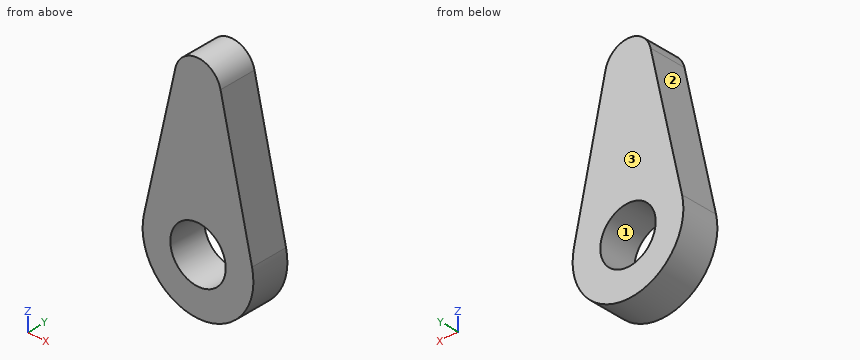
from build123d import *

# Parameters (mm, degrees)
F0_R     = 15
F1_DEPTH = 10


with BuildPart() as f1:
    # F0 (on Front) → F1 (new body, symmetric)
    with BuildSketch(Plane.XZ):
        with BuildLine():
            Line((-12.197262, 42.734375), (-29.273428, -33.4375))
            ThreePointArc((-29.273428, -33.4375), (0, -70), (29.273428, -33.4375))
            Line((29.273428, -33.4375), (12.197262, 42.734375))
            ThreePointArc((12.197262, 42.734375), (0, 52.5), (-12.197262, 42.734375))
        make_face()
        with Locations((0, -40)):
            Circle(F0_R, mode=Mode.SUBTRACT)
    extrude(amount=F1_DEPTH, both=True)


solid = f1.part
Model file for the job. Use its own axes, mm. Face numbers are marked on the shaded views. Coordinates: 2 decimals unless noted, no trailing zeros. Order: outer loops, then holes, each group sorted by start corner. A loop starts at its lowest first (then second) coordinate and runs counter-clockwise, first axis right, second up. Notation, with made-up numbers: M 85,-15.75 L 125,-15.75 A16 cw 125,-5.75 Z; hole C 38.5,-34 d7. An arc over 180 degrees is marked long. Return JSON: item names as keys, results as strings.
1. Saw through at A-A (x = 0). Give the cut face in (y, z), and give its area (3 significant figures).
Ans:
{"outline": "M -10,-70 L 10,-70 L 10,-55 L -10,-55 Z; M -10,-25 L 10,-25 L 10,52.5 L -10,52.5 Z", "area": "1,850 mm^2"}
2. Saw through at D-D (z = 10). Give the cut face in (x, y), and give its area (3 significant figures).
Ans:
{"outline": "M -19.54,-10 L 19.54,-10 L 19.54,10 L -19.54,10 Z", "area": "781 mm^2"}
3. Saw through at B-B (z = -40). Give the cut face in (x, y).
Ans:
{"outline": "M -30,-10 L -15,-10 L -15,10 L -30,10 Z; M 15,-10 L 30,-10 L 30,10 L 15,10 Z"}
4. Pull direction Z, two halves, no side cores. Call the marked faces 1, 2 and 3: +Z half, -Z half, draft (parallel to the pull), parting line (faces both ways), or undercut.
Ans:
{"face 1": "undercut", "face 2": "+Z half", "face 3": "draft"}
5. Flat gauge pins, fed straight in: pin 1 (1.5 mm diameter, centred on y = -3.5, z = -44, fed in from +X); pin 2 (1.5 mm diameter, centred on x = -21.5, y = -4.5, fed in from -Z); pin 3 (8 mm diameter, centred on y = -5.5, z = -20.5, fed in from +X). Where does each tip first touch, or does it go through?
Ans:
{"pin 1": "x = 29.82", "pin 2": "z = -61.67", "pin 3": "x = 27.27"}
6. Saw through at C-C (y = -2.75). Give the cut face in (x, z).
Ans:
{"outline": "M -29.27,-33.44 A30 ccw long 29.27,-33.44 L 12.2,42.73 A12.5 ccw -12.2,42.73 Z; hole C 0,-40 d30"}
7. Drill centre lines: probe 1 along Z at (x, y) = (0, -5.5); probe 2 along Z at (x, y) = (-7, -6.5); probe 3 along X at (y, z) = (-4.5, -41). Where is each one in solid material? Low to high.
Ans:
{"probe 1": "-70 to -55, -25 to 52.5", "probe 2": "-69.17 to -53.27, -26.73 to 50.36", "probe 3": "-29.98 to -14.97, 14.97 to 29.98"}
